Check sheet for the modelled part. Datum: model origin and axes. Units: mm. Round coordinates to 2 decimals unless told otherwise and drop trailing zeros. Order: outer loops, then holes, each group sorted by start corner. A loop starts at its lowest first (then second) coordinate and runs counter-clockwise, first axis right, second up. Notation, with made-up numbers: M 41.5,77.25 L 76.5,77.25 A12 cw 76.5,84.25 Z; hole C 9,67 d9. An arc over 180 degrees is marked long. One line per item, written item: value. Start each with the question number.
(1) Cross-section at D-D, the plane z = 82. Enter the section's corners in (x, y).
(2) Depth check by flat-ended pin: pin 1 Ø4 at (y, z) = (-25.5, 57.5) entering from +X; pin 2 Ø2 at (y, z) = (31.5, 119) entering from +X; pin 3 Ø5 at (x, y) = (-15.5, 36.5) entering from -Z; pin 4 Ø1 at (y, z) = (-38.5, 87.5) entering from +X. Enter the tip coordinate at first touch or a pass-through.
(3) Release check for a two-part mould opening along Z. For faces 1 (the face through (-1, -22, 150)), 2 (the face through (-1, -22, 0)), 3 (the face through (1, -23, 96.651)) record: released by +Z, released by -Z, zero draft, split by the parting line, or undercut.
(4) Cross-section at C-C, the plane z = 126. Enter the section's corners in (x, y).
(5) Cross-section at A-A, the plane y = 0. Enter the section's corners in (x, z), and give its area (3 significant figures).
(6) Thickness scan on L1, parallel to Y at x = 0, z = 24; L2, parallel to Z at x = -19, y = -18; L3, parallel to X at y = -38, z = 39. Record the ranges inside material, lowest first.
(7) Cross-section at B-B, the plane x = 32. Enter the section's corners in (y, z), and give its area (3 significant figures).
from build123d import *

# Parameters (mm, degrees)
F0_R     = 50
F1_DEPTH = 150
F2_R     = 21.443612
F3_DEPTH = 150.001
F5_DEPTH = 50.001
F6_DEPTH = 50.001


with BuildPart() as f1:
    # F0 (on Top) → F1 (new body)
    with BuildSketch(Plane.XY):
        Circle(F0_R)
    extrude(amount=F1_DEPTH)

    # F2 (on Top) → F3 (cut, through all)
    with BuildSketch(Plane.XY):
        Circle(F2_R)
    extrude(amount=F3_DEPTH, mode=Mode.SUBTRACT)

    # F4 (on Front) → F5 (cut, through all)
    with BuildSketch(Plane.XZ):
        Polygon((0, 96.650635), (0, 31.69873), (37.5, 96.650635), align=None)
        Polygon((-37.5, 96.650635), (0, 31.69873), (0, 96.650635), align=None)
    extrude(amount=F5_DEPTH, mode=Mode.SUBTRACT)

    # F4 (on Front) → F6 (cut, through all)
    with BuildSketch(Plane.XZ):
        Polygon((0, 96.650635), (0, 31.69873), (37.5, 96.650635), align=None)
        Polygon((-37.5, 96.650635), (0, 31.69873), (0, 96.650635), align=None)
    extrude(amount=-F6_DEPTH, mode=Mode.SUBTRACT)


solid = f1.part
Values found:
1. outline: M -29.04,-40.7 L -29.04,40.7 A50 ccw Z; M 29.04,-40.7 A50 ccw 29.04,40.7 Z
2. pin 1: x = 44.13
2. pin 2: x = 39.62
2. pin 3: z = 0
2. pin 4: x = 32.5
3. face 1: released by +Z
3. face 2: released by -Z
3. face 3: undercut
4. outline: C 0,0 d100; hole C 0,0 d42.89
5. outline: M -50,0 L -21.44,0 L -21.44,68.84 L -37.5,96.65 L -21.44,96.65 L -21.44,150 L -50,150 Z; M 21.44,0 L 50,0 L 50,150 L 21.44,150 L 21.44,96.65 L 37.5,96.65 L 21.44,68.84 Z
5. area: 8,120 mm^2
6. L1: -50 to -21.44, 21.44 to 50
6. L2: 0 to 64.61, 96.65 to 150
6. L3: -32.5 to -4.22, 4.22 to 32.5
7. outline: M -38.42,0 L 38.42,0 L 38.42,87.12 L -38.42,87.12 Z; M -38.42,96.65 L 38.42,96.65 L 38.42,150 L -38.42,150 Z
7. area: 10,800 mm^2
